from build123d import *

# Parameters (mm, degrees)
SKETCH2_W            = 820
SKETCH2_H            = 320
SKETCH2_W_2          = 750
SKETCH2_H_2          = 250
BOSS_EXTRUDE1_DEPTH  = 35
SKETCH7_W            = 35
SKETCH7_H            = 250
BOSS_EXTRUDE6_DEPTH  = 20
SKETCH3_W            = 35
SKETCH3_H            = 35
BOSS_EXTRUDE2_DEPTH  = 100
SKETCH4_W            = 820
SKETCH4_H            = 320
SKETCH4_W_2          = 750
SKETCH4_H_2          = 250
BOSS_EXTRUDE3_DEPTH  = 40
SKETCH5_W            = 35
SKETCH5_H            = 35
BOSS_EXTRUDE4_DEPTH  = 105
SHELL1_START         = -173.5
SHELL1_OUTLINE_W     = 817
SHELL1_OUTLINE_H     = 317
SHELL1_OUTLINE_W_2   = 753
SHELL1_OUTLINE_H_2   = 253
SHELL1_DEPTH         = 37
SHELL1_START_2       = -33.5
SHELL1_2_OUTLINE_W   = 817
SHELL1_2_OUTLINE_H   = 317
SHELL1_2_OUTLINE_W_2 = 753
SHELL1_2_OUTLINE_H_2 = 253
SHELL1_2_DEPTH       = 32
SHELL1_START_3       = -280
SHELL1_3_OUTLINE_W   = 32
SHELL1_3_OUTLINE_H   = 32
SHELL1_3_DEPTH       = 246.5
SHELL1_START_4       = -136.5
SHELL1_4_OUTLINE_W   = 32
SHELL1_4_OUTLINE_H   = 32
SHELL1_4_DEPTH       = 103
SHELL1_START_5       = -18.5
SHELL1_5_OUTLINE_W   = 32
SHELL1_5_OUTLINE_H   = 253
SHELL1_5_DEPTH       = 17
BOSS_EXTRUDE5_START  = 20
SKETCH6_R            = 8.5
BOSS_EXTRUDE5_DEPTH  = 48
SKETCH8_R            = 4
CUT_EXTRUDE1_DEPTH   = 30


# Read off the part's stored shape, not the designer's step: Shell1
with BuildPart() as part:
    # Sketch2 → Boss-Extrude1 (new body)
    with BuildSketch(Plane(origin=(0, 0, 0), x_dir=(1, 0, 0), z_dir=(0, 1, 0))):
        with Locations((410, 160)):
            Rectangle(SKETCH2_W, SKETCH2_H)
        with Locations((410, 160)):
            Rectangle(SKETCH2_W_2, SKETCH2_H_2, mode=Mode.SUBTRACT)
    extrude(amount=-BOSS_EXTRUDE1_DEPTH)

    # Sketch7 → Boss-Extrude6 (add)
    with BuildSketch(Plane(origin=(0, 0, 0), x_dir=(1, 0, 0), z_dir=(0, 1, 0))):
        with Locations((410, 160)):
            Rectangle(SKETCH7_W, SKETCH7_H)
    extrude(amount=-BOSS_EXTRUDE6_DEPTH)

    # Sketch3 → Boss-Extrude2 (add)
    with BuildSketch(Plane(origin=(0, -35, 0), x_dir=(-1, 0, 0), z_dir=(0, -1, 0))):
        with Locations((-17.5, 17.5)):
            Rectangle(SKETCH3_W, SKETCH3_H)
        with Locations((-17.5, 302.5)):
            Rectangle(SKETCH3_W, SKETCH3_H)
        with Locations((-802.5, 302.5)):
            Rectangle(SKETCH3_W, SKETCH3_H)
        with Locations((-802.5, 17.5)):
            Rectangle(SKETCH3_W, SKETCH3_H)
    extrude(amount=BOSS_EXTRUDE2_DEPTH)

    # Sketch4 → Boss-Extrude3 (add)
    with BuildSketch(Plane.XZ.offset(135)):
        with Locations((410, -160)):
            Rectangle(SKETCH4_W, SKETCH4_H)
        with Locations((410, -160)):
            Rectangle(SKETCH4_W_2, SKETCH4_H_2, mode=Mode.SUBTRACT)
    extrude(amount=BOSS_EXTRUDE3_DEPTH)

    # Sketch5 → Boss-Extrude4 (add)
    with BuildSketch(Plane.XZ.offset(175)):
        with Locations((802.5, -17.5)):
            Rectangle(SKETCH5_W, SKETCH5_H)
        with Locations((802.5, -302.5)):
            Rectangle(SKETCH5_W, SKETCH5_H)
    extrude(amount=BOSS_EXTRUDE4_DEPTH)

    # Shell1 outline → Shell1 (cut)
    with BuildSketch(Plane(origin=(0, 0, 0), x_dir=(1, 0, 0), z_dir=(0, 1, 0)).offset(SHELL1_START)):
        with Locations((410, 160)):
            Rectangle(SHELL1_OUTLINE_W, SHELL1_OUTLINE_H)
        with Locations((410, 160)):
            Rectangle(SHELL1_OUTLINE_W_2, SHELL1_OUTLINE_H_2, mode=Mode.SUBTRACT)
    extrude(amount=SHELL1_DEPTH, mode=Mode.SUBTRACT)

    # Shell1 2 outline → Shell1 2 (cut)
    with BuildSketch(Plane(origin=(0, 0, 0), x_dir=(1, 0, 0), z_dir=(0, 1, 0)).offset(SHELL1_START_2)):
        with Locations((410, 160)):
            Rectangle(SHELL1_2_OUTLINE_W, SHELL1_2_OUTLINE_H)
        with Locations((410, 160)):
            Rectangle(SHELL1_2_OUTLINE_W_2, SHELL1_2_OUTLINE_H_2, mode=Mode.SUBTRACT)
    extrude(amount=SHELL1_2_DEPTH, mode=Mode.SUBTRACT)

    # Shell1 3 outline → Shell1 3 (cut)
    with BuildSketch(Plane(origin=(0, 0, 0), x_dir=(1, 0, 0), z_dir=(0, 1, 0)).offset(SHELL1_START_3)):
        with Locations((802.5, 302.5)):
            Rectangle(SHELL1_3_OUTLINE_W, SHELL1_3_OUTLINE_H)
        with Locations((802.5, 17.5)):
            Rectangle(SHELL1_3_OUTLINE_W, SHELL1_3_OUTLINE_H)
    extrude(amount=SHELL1_3_DEPTH, mode=Mode.SUBTRACT)

    # Shell1 4 outline → Shell1 4 (cut)
    with BuildSketch(Plane(origin=(0, 0, 0), x_dir=(1, 0, 0), z_dir=(0, 1, 0)).offset(SHELL1_START_4)):
        with Locations((17.5, 302.5)):
            Rectangle(SHELL1_4_OUTLINE_W, SHELL1_4_OUTLINE_H)
        with Locations((17.5, 17.5)):
            Rectangle(SHELL1_4_OUTLINE_W, SHELL1_4_OUTLINE_H)
    extrude(amount=SHELL1_4_DEPTH, mode=Mode.SUBTRACT)

    # Shell1 5 outline → Shell1 5 (cut)
    with BuildSketch(Plane(origin=(0, 0, 0), x_dir=(1, 0, 0), z_dir=(0, 1, 0)).offset(SHELL1_START_5)):
        with Locations((410, 160)):
            Rectangle(SHELL1_5_OUTLINE_W, SHELL1_5_OUTLINE_H)
    extrude(amount=SHELL1_5_DEPTH, mode=Mode.SUBTRACT)

    # Sketch6 → Boss-Extrude5 (add)
    with BuildSketch(Plane(origin=(0, 0, 0), x_dir=(-1, 0, 0), z_dir=(0, -1, 0)).offset(BOSS_EXTRUDE5_START)):
        with Locations(Location((-410, 160, 0), (0, 0, 270))):
            Circle(SKETCH6_R)
    extrude(amount=BOSS_EXTRUDE5_DEPTH)

    # Sketch8 → Cut-Extrude1 (cut)
    with BuildSketch(Plane.XZ.offset(68)):
        with Locations(Location((410, -160, 0), (0, 0, 270))):
            Circle(SKETCH8_R)
    extrude(amount=-CUT_EXTRUDE1_DEPTH, mode=Mode.SUBTRACT)


solid = part.part
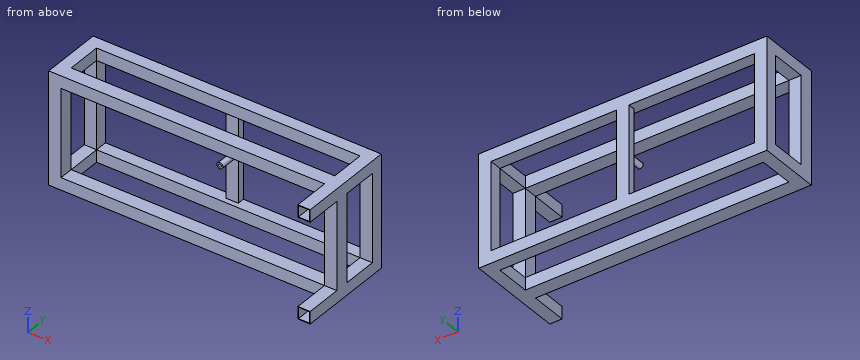
Input: part model. Units: mm. Frame: model coordinates. Round coordinates to 2 decimals unless told otherwise and drop trailing zeros. Loops run counter-clockwise (first coordinate to the right, second up) from the corner with the lowest first, then second, coordinate; pieces in that order, holes last. Notation, with made-up numbers: (39.25, 11.25) -> (84.25, 11.25) arc R17 ccw to (84.25, 34.25) -> close; hole circle Ø10 at (-23.5, -34). An arc over 180 degrees is marked (long way). Answer as a JSON object with one key per item and string values. Group by question number.
1) Section query C-C on z = -298.5. Output: boundary loops of the cut face in (x, y), plus the area to 3 significant figures.
2) Section query D-D on y = -154. Output: boundary loops of the cut face in (x, z), plus the area to 3 significant figures.
3) Pin query (flat end, axial travel): pin 1 (17.5 mm diameter, centred on x = 22, z = -159.5, fed in from -Y). Return the tip coordinate at first contact, or that it passes through.
4) Section query B-B on y = -259. Output: boundary loops of the cut face in (x, z), plus the area to 3 significant figures.
5) Section query A-A on x = 233. State how many separate pieces and enclosed holes the cut face has, plus the area to 3 significant figures.
6) Ray query, L1, parallel to X at y = -73.5, z = -28.5; L2, parallel to Z at x = 150.5, y = -13.5; L3, parallel to Y at x = 89.5, z = -31. Return the intervals inside material, ascending.
Reply:
{
 "1": {"outline": "(0, -175) -> (785, -175) -> (785, -280) -> (786.5, -280) -> (786.5, -173.5) -> (1.5, -173.5) -> (1.5, -1.5) -> (818.5, -1.5) -> (818.5, -280) -> (820, -280) -> (820, 0) -> (0, 0) -> close; (33.5, -136.5) -> (786.5, -136.5) -> (786.5, -33.5) -> (33.5, -33.5) -> close; hole (35, -135) -> (785, -135) -> (785, -35) -> (35, -35) -> close", "area": "5,800 mm2"},
 "2": {"outline": "(0, -320) -> (820, -320) -> (820, 0) -> (0, 0) -> close; (33.5, -286.5) -> (786.5, -286.5) -> (786.5, -33.5) -> (33.5, -33.5) -> close; hole (1.5, -318.5) -> (818.5, -318.5) -> (818.5, -1.5) -> (1.5, -1.5) -> close; hole (35, -285) -> (785, -285) -> (785, -35) -> (35, -35) -> close", "area": "6,420 mm2"},
 "3": {"pin 1": "stops at y = -175"},
 "4": {"outline": "(785, -320) -> (820, -320) -> (820, -285) -> (785, -285) -> close; (785, -35) -> (820, -35) -> (820, 0) -> (785, 0) -> close; hole (786.5, -318.5) -> (818.5, -318.5) -> (818.5, -286.5) -> (786.5, -286.5) -> close; hole (786.5, -33.5) -> (818.5, -33.5) -> (818.5, -1.5) -> (786.5, -1.5) -> close", "area": "402 mm2"},
 "5": {"separate pieces": "4", "enclosed holes": "4", "area": "834 mm2"},
 "6": {"L1": "x = 0 to 1.5, 33.5 to 35, 785 to 786.5, 818.5 to 820", "L2": "z = -320 to -318.5, -286.5 to -285, -35 to -33.5, -1.5 to 0", "L3": "y = -175 to -173.5, -136.5 to -135, -35 to -33.5, -1.5 to 0"}
}
